Could you check a few things on this model? Use its own coordinates, in mm. Face numbers are marked on the shaded views. A direction names the side the tool comes from. Round coordinates to 2 decimals unless told otherwise and drop trailing zeros. Order: outer loops, then holes, each group sorted by start corner. A loop starts at its lowest first (then second) coordinate and runs counter-clockwise, first axis right, second up. Notation, with made-up numbers: (-20.75, 13.25) -> (25.25, 13.25) arc R17 cw to (25.25, 28.25) -> close; hole circle Ø10 at (2.25, 27.5). An arc over 180 degrees is marked (long way). One line per question, with ' | ' between items.
```python
from build123d import *

# Parameters (mm, degrees)
SKETCH1_W      = 3.4036
SKETCH1_H      = 3.8862
EXTRUDE1_DEPTH = 16.764
EXTRUDE2_DEPTH = 0.6858
EXTRUDE3_DEPTH = 0.6858
EXTRUDE4_DEPTH = 1.27
SKETCH5_W      = 2.3876
SKETCH5_H      = 2.8702
EXTRUDE5_DEPTH = 9.906
SKETCH6_W      = 2.54
SKETCH6_H      = 2.54
EXTRUDE6_DEPTH = 6.35
EXTRUDE7_DEPTH = 9.906


with BuildPart() as part:
    # Sketch1 → Extrude1 (new body)
    with BuildSketch(Plane(origin=(0, 0, 0), x_dir=(0, 0, -1), z_dir=(1, 0, 0))):
        with Locations((-1.7018, 0)):
            Rectangle(SKETCH1_W, SKETCH1_H)
    extrude1 = extrude(amount=EXTRUDE1_DEPTH)

    # Sketch2 → Extrude2 (add)
    with BuildSketch(Plane(origin=(0, 1.9431, 0), x_dir=(1, 0, 0), z_dir=(0, 1, 0))):
        Polygon((0, -3.4036), (6.7564, -3.4036), (6.7564, -2.1336), (0.9906, -2.1336), (0.9906, -1.3716), (0, -1.3716), align=None)
    extrude2 = extrude(amount=EXTRUDE2_DEPTH)

    # Sketch3 → Extrude3 (add)
    with BuildSketch(Plane.XZ.offset(1.9431)):
        Polygon((0, 3.4036), (6.7564, 3.4036), (6.7564, 2.1336), (0.9906, 2.1336), (0.9906, 0), (0, 0), align=None)
    extrude3 = extrude(amount=EXTRUDE3_DEPTH)

    # Sketch4 → Extrude4 (add)
    with BuildSketch(Plane.XY):
        Polygon((16.4338, 1.9431), (14.9479, 3.0861), (14.1986, 3.0861), (14.1986, 1.9431), align=None)
    extrude4 = extrude(amount=EXTRUDE4_DEPTH)

    # Sketch5 → Extrude5 (cut)
    with BuildSketch(Plane(origin=(16.764, 0, 0), x_dir=(0, 0, -1), z_dir=(1, 0, 0))):
        with Locations((-1.7018, 0)):
            Rectangle(SKETCH5_W, SKETCH5_H)
    extrude5 = extrude(amount=-EXTRUDE5_DEPTH, mode=Mode.SUBTRACT)

    # Sketch6 → Extrude6 (cut)
    with BuildSketch(Plane.ZY):
        with Locations((1.4732, -0.0635)):
            Rectangle(SKETCH6_W, SKETCH6_H)
    extrude6 = extrude(amount=-EXTRUDE6_DEPTH, mode=Mode.SUBTRACT)

    # Mirror1: Extrude1, Extrude2, Extrude3, Extrude4, Extrude5, Extrude6 across Front Plane
    add(extrude1.mirror(Plane.XY))
    add(extrude2.mirror(Plane.XY))
    add(extrude3.mirror(Plane.XY))
    add(extrude4.mirror(Plane.XY))
    add(extrude5.mirror(Plane.XY), mode=Mode.SUBTRACT)
    add(extrude6.mirror(Plane.XY), mode=Mode.SUBTRACT)

    # Sketch7 → Extrude7 (add)
    with BuildSketch(Plane(origin=(6.858, 0, 0), x_dir=(0, 0, -1), z_dir=(1, 0, 0))):
        Polygon((0.508, -0.762663848), (1.033234934, -1.4351), (0.508, -1.4351), align=None)
    extrude(amount=EXTRUDE7_DEPTH)


solid = part.part
```
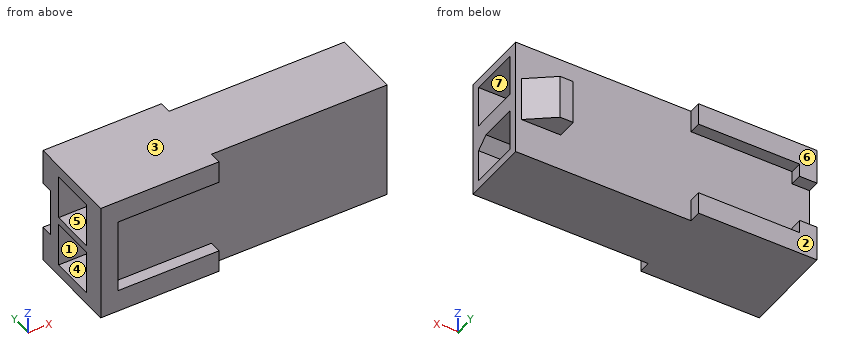
1. On a 3-axis mill with a long thin cutter (end or side, diameter ignored), from which of +Z, -Z, +X, -X, +Y, -Y can I reach the whole of each face in a straight line? I mean the marked faces 5, 6 and 7. Say none if no direction works.
From the geometry:
face 5: -X | face 6: +Z, -Z, +X, -X, +Y | face 7: +X
2. I need wall thicknesses on probe 1 along Z at (x, y) = (11, 0.45); probe 2 along Z at (x, y) = (4.75, -0.9); probe 3 along Y at (x, z) = (12.5, -1.25). Which ranges of each line are inside material? Lowest first, please.
From the geometry:
probe 1: z = -3.4 to -2.9, -0.51 to 0.51, 2.9 to 3.4 | probe 2: z = -3.4 to -2.74, -0.2 to 0.2, 2.74 to 3.4 | probe 3: y = -1.94 to -1.44, 1.44 to 1.94
3. I want a section at B-B on z = -2.5. List the corners of the cut face in (x, y) for me, and give its area (3 significant figures).
From the geometry:
outline: (0, -2.63) -> (6.76, -2.63) -> (6.76, -1.94) -> (16.76, -1.94) -> (16.76, -1.44) -> (6.86, -1.44) -> (6.86, 1.44) -> (16.76, 1.44) -> (16.76, 1.94) -> (6.76, 1.94) -> (6.76, 2.63) -> (0, 2.63) -> (0, 1.21) -> (6.35, 1.21) -> (6.35, -1.33) -> (0, -1.33) -> close | area: 29.9 mm²
4. I want a section at C-C on y = -0.5. List the corners of the cut face in (x, z) for me.
From the geometry:
outline: (0, -3.4) -> (16.76, -3.4) -> (16.76, -2.9) -> (6.86, -2.9) -> (6.86, -0.51) -> (16.76, -0.51) -> (16.76, 0.51) -> (6.86, 0.51) -> (6.86, 2.9) -> (16.76, 2.9) -> (16.76, 3.4) -> (0, 3.4) -> (0, 2.74) -> (6.35, 2.74) -> (6.35, 0.2) -> (0, 0.2) -> (0, -0.2) -> (6.35, -0.2) -> (6.35, -2.74) -> (0, -2.74) -> close
5. I'm going to push flat-ended pins straight in: pin 1 (1 mm diameter, centred on x = 2.5, z = 2, fed in from +Y); pin 2 (0.5 mm diameter, centred on y = -2.5, z = 2.5, fed in from +X); pin 3 (0.9 mm diameter, centred on x = 15, y = 2.5, fed in from +Z). Where does each tip first touch, or does it pass through?
From the geometry:
pin 1: stops at y = 2.63 | pin 2: stops at x = 6.76 | pin 3: stops at z = 1.27
6. If we mould it in two halves opening along Y, with no side actions, what happens to the marked faces 1, 2, 3 and 4? For each: pulls with the +Y half, pulls with the -Y half, needs draft (parallel to the pull), parting line crosses it, or undercut.
From the geometry:
face 1: undercut | face 2: pulls with the +Y half | face 3: needs draft | face 4: undercut
7. I want a section at D-D on x = 5.25. List the corners of the cut face in (y, z) for me.
From the geometry:
outline: (-2.63, -3.4) -> (2.63, -3.4) -> (2.63, -2.13) -> (1.94, -2.13) -> (1.94, 2.13) -> (2.63, 2.13) -> (2.63, 3.4) -> (-2.63, 3.4) -> (-2.63, 2.13) -> (-1.94, 2.13) -> (-1.94, -2.13) -> (-2.63, -2.13) -> close; hole (-1.33, -2.74) -> (1.21, -2.74) -> (1.21, -0.2) -> (-1.33, -0.2) -> close; hole (-1.33, 0.2) -> (1.21, 0.2) -> (1.21, 2.74) -> (-1.33, 2.74) -> close
8. I want a section at A-A on x = 9. List the corners of the cut face in (y, z) for me.
From the geometry:
outline: (-1.94, -3.4) -> (1.94, -3.4) -> (1.94, 3.4) -> (-1.94, 3.4) -> close; hole (-1.44, -2.9) -> (1.44, -2.9) -> (1.44, -0.51) -> (-0.76, -0.51) -> (-1.44, -1.03) -> close; hole (-1.44, 0.51) -> (1.44, 0.51) -> (1.44, 2.9) -> (-1.44, 2.9) -> close
